Read the model definition and answer for the solid it produces. Units are mm, in the model's axes. Face numbers are marked on the shaded views. A direction names the side the tool comes from. Give positions to 0.01 mm unless a question says otherwise; leave off trailing zeros. Write each loop counter-clockwise with the first axis right and the second up, starting at its lowest first coordinate (ties: lowest second). Pieces come first, ordered by that corner, then holes. Notation, with made-up numbers: (-37.5, -14) - (-26.5, -14) arc R12 cw to (-26.5, -8) - close; hole circle Ø3 at (18, 45). An arc over 180 degrees is marked (long way). Answer as CSV lines item,"result".
```python
from build123d import *

# Parameters (mm, degrees)
F0_R        = 9.5
F0_R_2      = 8
F1_DEPTH    = 2.5
F2_W        = 2.5811996311
F2_H        = 16.6603792459
F1_FACE_R   = 9.5
F1_FACE_R_2 = 8
F3_DEPTH    = 2.5
F0_R_3      = 4
F4_DEPTH    = 4
F7_START    = -20.3
F6_R        = 2.5
F7_DEPTH    = 4.7


with BuildPart() as f1:
    # F0 (on Front) → F1 (new body, symmetric)
    with BuildSketch(Plane.XZ):
        Circle(F0_R)
        Circle(F0_R_2, mode=Mode.SUBTRACT)
    extrude(amount=F1_DEPTH, both=True)

    # F2 (on Front) + F1_face (on face) → F3 (join)
    with BuildSketch(Plane.XZ):
        Rectangle(F2_W, F2_H)
    with BuildSketch(Plane(origin=(0, 2.5, 0), x_dir=(1, 0, 0), z_dir=(0, 1, 0))):
        Circle(F1_FACE_R)
        Circle(F1_FACE_R_2, mode=Mode.SUBTRACT)
    extrude(amount=F3_DEPTH, dir=(0, -1, 0))

    # F0 (on Front) → F4 (join)
    with BuildSketch(Plane.XZ):
        Circle(F0_R_2)
        Circle(F0_R_3, mode=Mode.SUBTRACT)
    extrude(amount=-F4_DEPTH)

    # F6 (on offset) → F7 (join)
    with BuildSketch(Plane(origin=(0, 25, 0), x_dir=(-1, 0, 0), z_dir=(0, 1, 0)).offset(F7_START)):
        Circle(F6_R)
    extrude(amount=-F7_DEPTH)


solid = f1.part
```
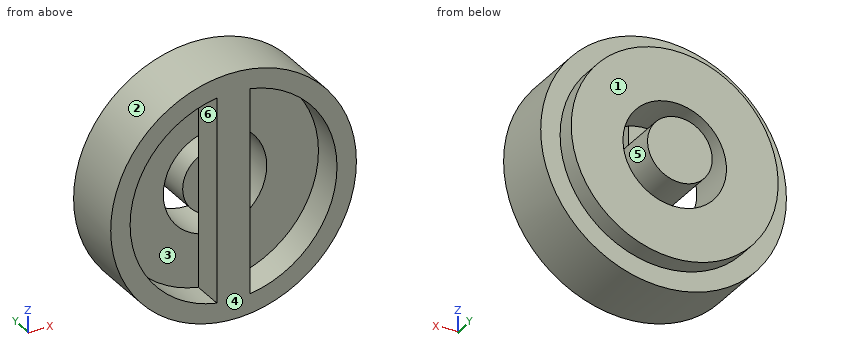
(1) For the marked faces 4, 5 and 6, determine the directions among +Z, -Z, +X, -X, +Y, -Y from which every point of the face is accessible in a straight line to the end or side of a thin tool.
Worked out:
face 4,"+Z, -Z, +X, -X, -Y"
face 5,"+Y"
face 6,"-Y"
(2) Each of these flat-tipped pins is pushed along its axis until it touches: P1, Ø0.8, axis at y = -0.5, z = -1, coming from the -X side; P2, Ø1.5, axis at y = 3, z = -3.5, coming from the -X side; P3, Ø0.9, axis at x = 0, z = 3.5, coming from the +Y side. Where does it stop, or does it pass through?
Worked out:
P1,"stops at x = -9.48"
P2,"stops at x = -9.03"
P3,"stops at y = 0"
(3) The mould has two halves that part along X. Classify the marked faces 1, 2 and 3: +X half, -X half, draft (parallel to the pull), parting line (faces both ways), or undercut.
Worked out:
face 1,"draft"
face 2,"parting line"
face 3,"undercut"
(4) A cutting plane is placed at A-A (y = -2). Write down the section's boundary in (x, z), and give its area (3 significant figures).
Worked out:
outline,"circle Ø19 at (0, 0); hole (-1.29, -7.9) - (-1.29, 7.9) arc R8 ccw to start; hole (1.29, -7.9) arc R8 ccw to (1.29, 7.9) - close"
area,"124 mm^2"
(5) A cutting plane is placed at D-D (x = 2.75). Write down the section's boundary in (y, z), and give its area (3 significant figures).
Worked out:
outline,"(-2.5, -9.09) - (2.5, -9.09) - (2.5, -7.51) - (4, -7.51) - (4, -2.9) - (0, -2.9) - (0, -7.51) - (-2.5, -7.51) - close; (-2.5, 7.51) - (0, 7.51) - (0, 2.9) - (4, 2.9) - (4, 7.51) - (2.5, 7.51) - (2.5, 9.09) - (-2.5, 9.09) - close"
area,"52.7 mm^2"
(6) A cutting plane is placed at B-B (z = 0). Write down the section's boundary in (x, y), and give its area (3 significant figures).
Worked out:
outline,"(-9.5, -2.5) - (-8, -2.5) - (-8, 0) - (-4, 0) - (-4, 4) - (-8, 4) - (-8, 2.5) - (-9.5, 2.5) - close; (-2.5, 0) - (-1.29, 0) - (-1.29, -2.5) - (1.29, -2.5) - (1.29, 0) - (2.5, 0) - (2.5, 4.7) - (-2.5, 4.7) - close; (4, 0) - (8, 0) - (8, -2.5) - (9.5, -2.5) - (9.5, 2.5) - (8, 2.5) - (8, 4) - (4, 4) - close"
area,"77.0 mm^2"
(7) A cutting plane is placed at C-C (x = 0). Write down the section's boundary in (y, z).
Worked out:
outline,"(-2.5, -9.5) - (2.5, -9.5) - (2.5, -8) - (4, -8) - (4, -4) - (0, -4) - (0, -2.5) - (4.7, -2.5) - (4.7, 2.5) - (0, 2.5) - (0, 4) - (4, 4) - (4, 8) - (2.5, 8) - (2.5, 9.5) - (-2.5, 9.5) - close"
(8) Find the intervals of material crossed by L1, parallel to Z at x = 0, y = 3.1; L2, parallel to Z at x = 0, y = 0.8; L3, parallel to X at y = -1.5, z = 5.75, in increasing order.
Worked out:
L1,"z = -8 to -4, -2.5 to 2.5, 4 to 8"
L2,"z = -9.5 to -4, -2.5 to 2.5, 4 to 9.5"
L3,"x = -7.56 to -5.56, -1.29 to 1.29, 5.56 to 7.56"
